The listing builds one solid part. Answer for the finished solid, in the listing's coordinates (mm). A direction names the side the tool comes from. Give positions to 0.01 mm unless a question says otherwise; leave off trailing zeros. Order: outer loops, then holes, each group sorted by start corner. A loop starts at its lowest first (then second) coordinate and runs counter-clockwise, first axis right, second up.
```python
from build123d import *

# Parameters (mm, degrees)
SKETCH1_W           = 6.35
SKETCH1_H           = 1.996855346
SKETCH2_R           = 5.5
BOSS_EXTRUDE1_DEPTH = 23.5
CUT_EXTRUDE1_DEPTH  = 10
FILLET1_R           = 0.5


with BuildPart() as part:
    # Sketch1 → Revolve1 (revolve)
    with BuildSketch(Plane(origin=(0, 0, 0), x_dir=(-1, 0, 0), z_dir=(0, 0, -1)), mode=Mode.PRIVATE) as revolve1_sk:
        with Locations((-3.175, 0.998427673)):
            Rectangle(SKETCH1_W, SKETCH1_H)
    revolve(revolve1_sk.sketch.rotate(Axis((0, 0, 0), (0, 1, 0)), 270), axis=Axis((0, 0, 0), (0, 1, 0)))

    # Sketch2 → Boss-Extrude1 (add)
    with BuildSketch(Plane.XZ):
        with Locations(Location((0, 0, 0), (0, 0, 270))):
            Circle(SKETCH2_R)
    extrude(amount=BOSS_EXTRUDE1_DEPTH)

    # Sketch3 → Cut-Extrude1 (cut)
    with BuildSketch(Plane(origin=(0, 1.996855346, 0), x_dir=(-1, 0, 0), z_dir=(0, 1, 0))):
        with BuildLine():
            ThreePointArc((1.75, 0), (1.686558319, 0.466927227), (1.500833102, 0.9))
            Line((1.500833102, 0.9), (-1.500833102, 0.9))
            Line((-1.500833102, 0.9), (-1.500833102, 0))
            Line((-1.500833102, 0), (1.75, 0))
        make_face()
        with BuildLine():
            Line((4.499166898, 0), (4.499166898, 0.9))
            Line((4.499166898, 0.9), (1.500833102, 0.9))
            ThreePointArc((1.500833102, 0.9), (1.686558319, 0.466927227), (1.75, 0))
            Line((1.75, 0), (4.499166898, 0))
        make_face()
        with BuildLine():
            Line((4.499166898, -0.9), (4.499166898, 0))
            Line((4.499166898, 0), (1.75, 0))
            ThreePointArc((1.75, 0), (1.686558319, -0.466927227), (1.500833102, -0.9))
            Line((1.500833102, -0.9), (4.499166898, -0.9))
        make_face()
        with BuildLine():
            ThreePointArc((1.500833102, -0.9), (1.686558319, -0.466927227), (1.75, 0))
            Line((1.75, 0), (-1.500833102, 0))
            Line((-1.500833102, 0), (-1.500833102, -0.9))
            ThreePointArc((-1.500833102, -0.9), (-1.373979193, -1.083827098), (-1.224744871, -1.25))
            Line((-1.224744871, -1.25), (1.224744871, -1.25))
            ThreePointArc((1.224744871, -1.25), (1.373979193, -1.083827098), (1.500833102, -0.9))
        make_face()
    extrude(amount=-CUT_EXTRUDE1_DEPTH, mode=Mode.SUBTRACT)

    # Fillet1
    fillet1_edges = [part.edges().sort_by_distance(p)[0] for p in [
        (0, 1.996855346, -6.35),
    ]]
    fillet(fillet1_edges, radius=FILLET1_R)

    # Cut-Extrude2 cone 1 section (on through the dimple's axis) → Cut-Extrude2 (revolve, cut)
    with BuildSketch(Plane(origin=(0, 1.996855346, 0), x_dir=(0, 0, 1), z_dir=(1, 0, 0))):
        Polygon((0, 0), (1.75, 0), (0, 1.75), align=None)
    revolve(axis=Axis((0, 1.996855346, 0), (0, -1, 0)), mode=Mode.SUBTRACT)


solid = part.part
```
1) Find section B-B (x = 0). Write down the section's boundary in (y, z).
Geometry says:
outline: (-23.5, -5.5) - (0, -5.5) - (0, -6.35) - (1.5, -6.35) arc R0.5 ccw to (2, -5.85) - (2, -1.75) - (1.5, -1.25) - (-8, -1.25) - (-8, 0.9) - (1.15, 0.9) - (2, 1.75) - (2, 5.85) arc R0.5 ccw to (1.5, 6.35) - (0, 6.35) - (0, 5.5) - (-23.5, 5.5) - close
2) Find section A-A (y = 0.5). Write down the section's boundary in (x, z), then the cut area to 3 significant figures.
Geometry says:
outline: circle Ø12.7 at (0, 0); hole (-4.5, -0.9) - (-1.5, -0.9) arc R1.75 ccw to (-1.22, -1.25) - (1.22, -1.25) arc R1.75 ccw to (1.5, -0.9) - (1.5, 0.9) - (-4.5, 0.9) - close
area: 115 mm2
3) A tool of negligible diameter and unlimited length cuts with its end or side. For faces 1 (the flat face through (-2, -3, 0.9)), 2 (the flat face through (1.4, 1.997, -1.4)), 3 (the flat face through (3, 0, -5)), from which of +Z, -Z, +X, -X, +Y, -Y can it reach the whole face along a straight path? Write none if from no direction.
Geometry says:
face 1: +Y
face 2: +Z, -Z, +X, -X, +Y
face 3: -Y
4) Straight lines are drawn through the part: probe 1 along X at (y, z) = (-3.5, 0); probe 2 along Y at (x, z) = (1.25, 5.5); probe 3 along Z at (x, y) = (-0.5, -3). For each, find the intervals that lie inside material, in ascending order.
Geometry says:
probe 1: x = -5.5 to -4.5, 1.5 to 5.5
probe 2: y = 0 to 2
probe 3: z = -5.48 to -1.25, 0.9 to 5.48
5) Find section D-D (y = -5). Write down the section's boundary in (x, z).
Geometry says:
outline: circle Ø11 at (0, 0); hole (-4.5, -0.9) - (-1.5, -0.9) arc R1.75 ccw to (-1.22, -1.25) - (1.22, -1.25) arc R1.75 ccw to (1.5, -0.9) - (1.5, 0.9) - (-4.5, 0.9) - close
6) Find section C-C (z = 0). Write down the section's boundary in (x, y).
Geometry says:
outline: (-6.35, 0) - (-5.5, 0) - (-5.5, -23.5) - (5.5, -23.5) - (5.5, 0) - (6.35, 0) - (6.35, 1.5) arc R0.5 ccw to (5.85, 2) - (1.75, 2) - (1.5, 1.75) - (1.5, -8) - (-4.5, -8) - (-4.5, 2) - (-5.85, 2) arc R0.5 ccw to (-6.35, 1.5) - close
7) For a pull along X with two mould halves and no side action, classify faces 4 (the cylindrical face through (-5.37, -11.59, 1.19)), 5 (the flat face through (-4.499, -3, 0)), 6 (the flat face through (0, -23.5, 0)) as +X half, -X half, draft (parallel to the pull), parting line (faces both ways), or undercut.
Geometry says:
face 4: parting line
face 5: undercut
face 6: draft
8) Given P1, Ø1.5, axis at x = 4, y = -19.5, coming from the -Z side; P2, Ø5, axis at x = -0.5, y = -4, coming from the -Z side; P3, Ø1, axis at y = -15, z = -0.5, coming from the +X side, each flat-ended and moving along its own axis, determine where each tip first touches the part or whether it passes through.
Geometry says:
P1: stops at z = -4.44
P2: stops at z = -5.5
P3: stops at x = 5.5
